Autodesk Inventor part; units mm, degrees
ref_plane "YZ Plane" through (0, 0, 0) normal (1, 0, 0) x (0, 1, 0)
ref_plane "XZ Plane" through (0, 0, 0) normal (0, 1, 0) x (-1, 0, 0)
ref_plane "XY Plane" through (0, 0, 0) normal (0, 0, 1) x (1, 0, 0)
sketch "Sketch12" plane through (0, 0, 0) normal (0, 1, 0) x (-1, 0, 0)
  line L0 (0, 0) -> (0, 40)
  line L1 (0, 40) -> (80, 40)
  line L2 (80, 40) -> (80, 0)
  line L3 (80, 0) -> (80, -40)
  line L4 (80, -40) -> (0, -40)
  line L5 (0, -40) -> (0, 0)
  dimension "d39" = 40
  dimension "d40" = 80
  dimension "d41" = 40
extrude "Extrusion10" add sketch "Sketch12" along normal blind 40
shell "Shell2" thickness 1 removed faces 2 at (-26.6667, 0, -13.3333) at (-26.6667, 40, -13.3333)
sketch "Sketch13" plane through (-80, 0, -40) normal (-1, 0, 0) x (0, 0, 1)
  line L0 (0, 0) -> (80, 0)
  line L1 (80, 40) -> (0, 40)
  circle A0 centre (40, 20) radius 3.5
  point P0 (40, 0)
  dimension "d45" = 7
extrude "Extrusion11" cut sketch "Sketch13" against normal blind 1
properties part number "MAN_BASIS_PRIMARY_STRUCTURE" material "ABS Plastic"
Part model, mm, in its own coordinate system. A direction names the side the tool comes from. Give positions to 0.01 mm unless a question says otherwise; leave off trailing zeros. Order: outer loops, then holes, each group sorted by start corner. A loop starts at its lowest first (then second) coordinate and runs counter-clockwise, first axis right, second up. Notation, with made-up numbers: M 51,-25 L 63,-25 A13 ccw 63,-3 Z; hole C 85.25,40 d3. An arc over 180 degrees is marked long. Use a Markdown table: item, result. Add a question column.
(1) Mould opens along Z. For faces 1 (the face through (-41, 20, -39)), 2 (the face through (-39, 20, 40)), 3 (the face through (0, 20, -1)) say: +Z half, -Z half, draft (parallel to the pull), parting line (faces both ways), or undercut.
(2) Saw through at A-A, the plane x = -10. Give the cut face in (y, z).
(3) Saw through at C-C, the plane y = 20. Give the cut face in (x, z), and give its area (3 significant figures).
(4) Probe line 1 along Y through (x, z) = (-79.25, 0); line 2 along Z through (x, y) = (-79.5, 20); line 3 along Z through (x, y) = (-68.5, 9). List the from-to ranges inside material, lowest first. Write a range as [from, to].
(5) Drop a flat-ended pin along its axis: P1, Ø20, axis at y = 18.5, z = 1.5, coming from the -X side. Give the stop position or say it passes through.
(6) Saw through at B-B, the plane z = 0. Give the cut face in (x, y).
(7) Saw through at D-D, the plane z = -25. Give the cut face in (x, y).
(8) 3-axis set-ups, long thin cutter, end or side, ignore diameter. For faces 4 (the face through (-39, 20, 39)), 5 (the face through (-79.51, 23.47, -0.46)), 6 (the face through (-80, 24, 1)): which of +Z, -Z, +X, -X, +Y, -Y reach the whole face in a straight line?
Answer key:
| question | item | result |
|---|---|---|
| 1 | face 1 | undercut |
| 1 | face 2 | +Z half |
| 1 | face 3 | draft |
| 2 | outline | M 0,-40 L 40,-40 L 40,-39 L 0,-39 Z; M 0,39 L 40,39 L 40,40 L 0,40 Z |
| 3 | outline | M -80,-40 L 0,-40 L 0,40 L -80,40 L -80,3.5 L -79,3.5 L -79,39 L -1,39 L -1,-39 L -79,-39 L -79,-3.5 L -80,-3.5 Z |
| 3 | area | 309 mm^2 |
| 4 | line 1 | [0, 16.5], [23.5, 40] |
| 4 | line 2 | [-40, -3.5], [3.5, 40] |
| 4 | line 3 | [-40, -39], [39, 40] |
| 5 | P1 | x = -80 |
| 6 | outline | M -80,0 L -79,0 L -79,16.5 L -80,16.5 Z; M -80,23.5 L -79,23.5 L -79,40 L -80,40 Z; M -1,0 L 0,0 L 0,40 L -1,40 Z |
| 7 | outline | M -80,0 L -79,0 L -79,40 L -80,40 Z; M -1,0 L 0,0 L 0,40 L -1,40 Z |
| 8 | face 4 | +Y, -Y |
| 8 | face 5 | -X |
| 8 | face 6 | +Z, -Z, -X, +Y, -Y |
